from build123d import *

# Parameters (mm, degrees)
F0_R     = 78.74
F0_R_2   = 4.208
F0_R_3   = 4.2080161266
F1_DEPTH = 5.17
F3_DEPTH = 3
F4_R     = 1.5
F5_DEPTH = 25


# Not quite as in the source:
# - a feature names something its author has since deleted; it is built from what else it names


with BuildPart() as f1:
    # F0 (on Top) → F1 (new body)
    with BuildSketch(Plane.XY):
        with Locations((-0.1257307514, 0.2739626218)):
            Circle(F0_R)
        with Locations((-49.0250116127, -49.6047185081)):
            Circle(F0_R_2, mode=Mode.SUBTRACT)
        with Locations((49.0554707364, -49.3247707953)):
            Circle(F0_R_3, mode=Mode.SUBTRACT)
        with Locations((-49.7306512766, 49.450932452)):
            Circle(F0_R_2, mode=Mode.SUBTRACT)
        with BuildLine():
            ThreePointArc((41.6625381497, 44.7120159348), (49.6362217188, 35.5549502263), (55.6382636856, 25))
            Line((55.6382636856, 25), (70.6142692486, 25))
            Line((70.6142692486, 25), (70.6142692486, -25))
            Line((70.6142692486, -25), (55.3920755218, -25))
            ThreePointArc((55.3920755218, -25), (49.182592498, -35.6382812281), (40.9624707364, -44.8121738117))
            Line((40.9624707364, -44.8121738117), (40.9624707364, -63.790228106))
            Line((40.9624707364, -63.790228106), (21.9624707364, -63.790228106))
            Line((21.9624707364, -63.790228106), (21.9624707364, -56.5864924857))
            ThreePointArc((21.9624707364, -56.5864924857), (17.2267771251, -58.2058669812), (12.3742692486, -59.4315647605))
            Line((12.3742692486, -59.4315647605), (12.3742692486, -71.9660373782))
            Line((12.3742692486, -71.9660373782), (-12.6257307514, -71.9660373782))
            Line((-12.6257307514, -71.9660373782), (-12.6257307514, -74.9675166541))
            ThreePointArc((-12.6257307514, -74.9675166541), (-27.09160778, -71.308076376), (-40.5250116127, -64.8121728344))
            Line((-40.5250116127, -64.8121728344), (-40.5250116127, -45.4305022137))
            ThreePointArc((-40.5250116127, -45.4305022137), (-61.1238878157, -0.2002048119), (-41.2306512766, 45.3448568731))
            Line((-41.2306512766, 45.3448568731), (-41.2306512766, 64.9332740284))
            ThreePointArc((-41.2306512766, 64.9332740284), (-27.3884909599, 71.6521165865), (-12.5, 75.5355537871))
            Line((-12.5, 75.5355537871), (-12.5, 72.5138622393))
            Line((-12.5, 72.5138622393), (0, 72.5138622393))
            Line((0, 72.5138622393), (12.5, 72.5138622393))
            Line((12.5, 72.5138622393), (12.5, 59.9530286583))
            ThreePointArc((12.5, 59.9530286583), (17.6487859305, 58.6269107626), (22.6625381497, 56.8574831953))
            Line((22.6625381497, 56.8574831953), (22.6625381497, 63.8574831953))
            Line((22.6625381497, 63.8574831953), (41.6625381497, 63.8574831953))
            Line((41.6625381497, 63.8574831953), (41.6625381497, 44.7120159348))
        make_face(mode=Mode.SUBTRACT)
        with Locations((49.75511293, 49.1690173001)):
            Circle(F0_R_2, mode=Mode.SUBTRACT)
    extrude(amount=F1_DEPTH)

    # F2 (on face) → F3 (cut)
    with BuildSketch(Plane(origin=(0, 0, 0), x_dir=(1, 0, 0), z_dir=(0, 0, -1))):
        with BuildLine():
            ThreePointArc((-22.6257307514, 75.1828965761), (-28.7215245435, 73.0899806842), (-34.6257307514, 70.5055372352))
            Line((-34.6257307514, 70.5055372352), (-34.6257307514, 68.081065471))
            ThreePointArc((-34.6257307514, 68.081065471), (-28.7284061022, 70.69020135), (-22.6257307514, 72.7742794712))
            Line((-22.6257307514, 72.7742794712), (-22.6257307514, 75.1828965761))
        make_face()
        with BuildLine():
            Line((-34.5, -68.6212157755), (-34.5, -71.1146092424))
            ThreePointArc((-34.5, -71.1146092424), (-28.5952430236, -73.6870028189), (-22.5, -75.7681986639))
            Line((-22.5, -75.7681986639), (-22.5, -73.2755617719))
            ThreePointArc((-22.5, -73.2755617719), (-28.595756362, -71.1952712241), (-34.5, -68.6212157755))
        make_face()
        with BuildLine():
            ThreePointArc((-49.5286609465, -36.0559481471), (-52.707319331, -31.1960670528), (-55.4094464584, -26.0559481471))
            Line((-55.4094464584, -26.0559481471), (-74.5251717599, -26.0559481471))
            ThreePointArc((-74.5251717599, -26.0559481471), (-72.5682702123, -31.1295306193), (-70.2658555864, -36.0559481471))
            Line((-70.2658555864, -36.0559481471), (-49.5286609465, -36.0559481471))
        make_face()
        with BuildLine():
            ThreePointArc((-60.8510849569, -6.0559481471), (-61.1253373513, -0.0548857934), (-60.807987598, 5.9440518529))
            Line((-60.807987598, 5.9440518529), (-78.6198317781, 5.9440518529))
            ThreePointArc((-78.6198317781, 5.9440518529), (-78.86542717, -0.0553124259), (-78.6531542631, -6.0559481471))
            Line((-78.6531542631, -6.0559481471), (-60.8510849569, -6.0559481471))
        make_face()
        with BuildLine():
            ThreePointArc((-55.2039997602, 25.9440518529), (-52.4464078958, 31.0875861785), (-49.2098975215, 35.9440518529))
            Line((-49.2098975215, 35.9440518529), (-70.0417019419, 35.9440518529))
            ThreePointArc((-70.0417019419, 35.9440518529), (-72.3803771023, 31.0190666452), (-74.3726385456, 25.9440518529))
            Line((-74.3726385456, 25.9440518529), (-55.2039997602, 25.9440518529))
        make_face()
        with BuildLine():
            Line((2.5, -72.5138622393), (2.5, -78.9701705229))
            ThreePointArc((2.5, -78.9701705229), (7.5155682015, -78.6423117834), (12.5, -77.9951214075))
            Line((12.5, -77.9951214075), (12.5, -72.5138622393))
            Line((12.5, -72.5138622393), (2.5, -72.5138622393))
        make_face()
        with BuildLine():
            ThreePointArc((12.3742692486, 77.4675166541), (7.3895759923, 78.1065691737), (2.3742692486, 78.4263397919))
            Line((2.3742692486, 78.4263397919), (2.3742692486, 71.9660373782))
            Line((2.3742692486, 71.9660373782), (12.3742692486, 71.9660373782))
            Line((12.3742692486, 71.9660373782), (12.3742692486, 77.4675166541))
        make_face()
        with BuildLine():
            ThreePointArc((20.3742692486, 75.7506228753), (17.8838503139, 76.3787776414), (15.3742692486, 76.9253741629))
            Line((15.3742692486, 76.9253741629), (15.3742692486, 58.7239186961))
            ThreePointArc((15.3742692486, 58.7239186961), (17.8908537815, 58.0047014138), (20.3742692486, 57.1781913848))
            Line((20.3742692486, 57.1781913848), (20.3742692486, 75.7506228753))
        make_face()
        with BuildLine():
            Line((15.5, -59.238668493), (15.5, -77.4479487731))
            ThreePointArc((15.5, -77.4479487731), (18.0096554679, -76.8970359527), (20.5, -76.2645332932))
            Line((20.5, -76.2645332932), (20.5, -57.6810983365))
            ThreePointArc((20.5, -57.6810983365), (18.0167228167, -58.5135658015), (15.5, -59.238668493))
        make_face()
        with BuildLine():
            ThreePointArc((66.3344029178, -42.5), (70.5632346959, -34.9590857149), (73.9398248467, -27))
            Line((73.9398248467, -27), (54.7078258181, -27))
            ThreePointArc((54.7078258181, -27), (49.9060787318, -35.1712123678), (43.8965564147, -42.5))
            Line((43.8965564147, -42.5), (66.3344029178, -42.5))
        make_face()
        with BuildLine():
            ThreePointArc((73.7398130624, 27), (70.2892388263, 34.9640801641), (65.9830865246, 42.5))
            Line((65.9830865246, 42.5), (43.3643614724, 42.5))
            ThreePointArc((43.3643614724, 42.5), (49.5096317795, 35.1848978566), (54.4373608299, 27))
            Line((54.4373608299, 27), (73.7398130624, 27))
        make_face()
    extrude(amount=-F3_DEPTH, mode=Mode.SUBTRACT)

    # F4 (on face) → F5 (cut)
    with BuildSketch(Plane(origin=(0, 0, 3), x_dir=(1, 0, 0), z_dir=(0, 0, -1))):
        with Locations((-74.5251700282, 0)):
            Circle(F4_R)
        with Locations((-59.8972582664, 30.7893175632)):
            Circle(F4_R)
        with Locations((-59.8972582664, -31.6777378321)):
            Circle(F4_R)
        with Locations((8.0563814701, -75.5707131466)):
            Circle(F4_R)
        with Locations((6.9561954952, 75.5563961955)):
            Circle(F4_R)
        with Locations((58.2362919726, 35.7437855263)):
            Circle(F4_R)
        with Locations((58.4940314293, -36.4654541612)):
            Circle(F4_R)
    extrude(amount=-F5_DEPTH, mode=Mode.SUBTRACT)


solid = f1.part
Verification items for the finished model (mm, model axes). A direction names the side the tool comes from. Give positions to 0.01 mm unless a question says otherwise; leave off trailing zeros. Write each loop counter-clockwise with the first axis right and the second up, starting at its lowest first coordinate (ties: lowest second). Pieces come first, ordered by that corner, then holes. Notation, with made-up numbers: M -33,43.25 L -9,43.25 A14 ccw -9,61.25 Z; hole C 15.5,-39.5 d9. An arc over 180 degrees is marked long. Put each result on its own line as item: value. Start each with the question number.
1. Section check B-B (y = 12). Record the cut outline in (x, z).
2. Go/stop test with flat-tipped pins: pin 1 Ø3 at (x, y) = (5, -76.5) entering from -Z; pin 2 Ø3 at (y, z) = (-12.5, 3.5) entering from -X; pin 3 Ø2.5 at (x, z) = (0, 3) entering from -Y; pin 4 Ø1 at (x, z) = (-30.5, 1.5) entering from -Y. Record where each tip stops, or that it passes through.
3. Section check A-A (x = -37.5). Record the cut outline in (y, z), and give its area (3 significant figures).
4. Scan lines: line 1 along Y through (x, z) = (69, 1); line 2 along Y through (x, z) = (57.5, 4.35); line 3 along Y through (x, z) = (-54, 2.3). Record each from-to range of solid material in increasing order. Write a range as [from, to].
5. Section check C-C (z = 2). Give the number of separate pieces and of enclosed holes in the cut face, and give its area (3 significant figures).
6. Draft check along Y on faces 5 (the face through (41.4, -59, 0)), 6 (the face through (-26.89, -71.38, 3.7)), 7 (the face through (42.2, 66.67, 2.55)). Enter one of: +Y half, -Y half, draft (parallel to the pull), parting line (faces both ways), or undercut.
7. Set-up check for faces 1 (the face through (58.7, 34.6, 3)), 2 (the face through (-53, 46, 0)), 3 (the face through (17.578, 58.649, 3.698)), 4 (the face through (12.374, -66, 3)): record each of +Z, -Z, +X, -X, +Y, -Y from which the full face is reachable in a straight line by a thin tool's end or side.
Answer list:
1. outline: M -77.99,0 L -59.99,0 L -59.99,5.17 L -77.99,5.17 Z; M 70.61,0 L 77.74,0 L 77.74,5.17 L 70.61,5.17 Z
2. pin 1: z = 3
2. pin 2: x = -78.05
2. pin 3: y = -78.47
2. pin 4: through
3. outline: M -69.03,0 L -66.58,0 L -66.58,5.17 L -69.03,5.17 Z; M 67.08,0 L 69.58,0 L 69.58,5.17 L 67.08,5.17 Z
3. area: 25.6 mm2
4. line 1: [-27, -25], [25, 27]
4. line 2: [-53.38, -37.05], [-34.44, -25], [25, 35.34], [37.59, 53.93]
4. line 3: [-57.15, -35.94], [36.06, 57.7]
5. separate pieces: 11
5. enclosed holes: 4
5. area: 3,360 mm2
6. face 5: draft
6. face 6: undercut
6. face 7: parting line
7. face 1: -Z, +X
7. face 2: -Z, +X, -X, +Y, -Y
7. face 3: +Z, -Z
7. face 4: -Z
